```python
from build123d import *

# Parameters (mm, degrees)
CYLINDER_R           = 1.75
CYLINDER_DEPTH       = 10
CYLINDER001_R        = 4.25
CYLINDER001_DEPTH    = 8
CLONE001_ROLL_ANGLE  = 90
CLONE001_PITCH_ANGLE = -45


with BuildPart() as spacer_hole_cylinder:
    # Cylinder → Cylinder (new body)
    with BuildSketch(Plane.XY.offset(-1)):
        Circle(CYLINDER_R)
    extrude(amount=CYLINDER_DEPTH)


with BuildPart() as x_motor_spacer_top:
    # Cylinder001 → Cylinder001 (new body)
    with BuildSketch(Plane.XY):
        Circle(CYLINDER001_R)
    extrude(amount=CYLINDER001_DEPTH)

    # Cut002: cut spacer-hole-cylinder
    add(spacer_hole_cylinder.part, mode=Mode.SUBTRACT)


with BuildPart() as x_motor_spacer_top_1:
    # Clone001 roll: moved
    add(x_motor_spacer_top.part.rotate(Axis((0, 0, 0), (1, 0, 0)), CLONE001_ROLL_ANGLE))


with BuildPart() as x_motor_spacer_top_2:
    # Clone001 pitch: moved
    add(x_motor_spacer_top_1.part.rotate(Axis((0, 0, 0), (0, 1, 0)), CLONE001_PITCH_ANGLE))


with BuildPart() as x_motor_spacer_top_3:
    # Clone001 placement: moved
    add(x_motor_spacer_top_2.part.moved(Location((-49.5, 1, 41.384776))))


solid = x_motor_spacer_top_3.part
```
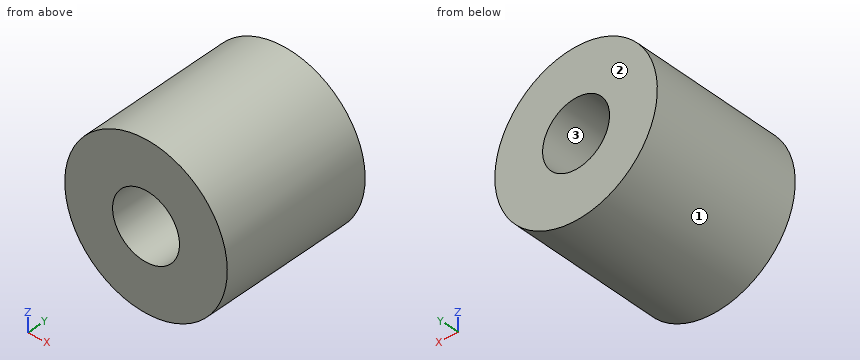
Read the model definition and answer for the solid it produces. Units are mm, in the model's axes. Face numbers are marked on the shaded views. Coordinates: 2 decimals unless noted, no trailing zeros. Loops run counter-clockwise (first coordinate to the right, second up) from the corner with the lowest first, then second, coordinate; pieces in that order, holes last. Notation, with made-up numbers: (34, -24) - (45, -24) arc R29 cw to (45, 6) - close; hole circle Ø5 at (86, 82). An arc over 180 degrees is marked (long way). Answer in a Markdown table with one row per item.
1. Find section A-A, the plane x = -49.5. Write down the section's boundary in (y, z).
Conclusion:
| item | result |
|---|---|
| outline | (-7, 37.13) - (1, 37.13) - (1, 39.63) - (-7, 39.63) - close; (-7, 43.13) - (1, 43.13) - (1, 45.63) - (-7, 45.63) - close |
2. Find section C-C, the plane y = -0.5. Write down the section's boundary in (x, z), then the cut area to 3 significant figures.
Conclusion:
| item | result |
|---|---|
| outline | circle Ø8.5 at (-49.5, 41.38); hole circle Ø3.5 at (-49.5, 41.38) |
| area | 47.1 mm² |
3. Find section B-B, the plane x = -51. Write down the section's boundary in (y, z), then the cut area to 3 significant figures.
Conclusion:
| item | result |
|---|---|
| outline | (-7, 37.41) - (1, 37.41) - (1, 40.48) - (-7, 40.48) - close; (-7, 42.29) - (1, 42.29) - (1, 45.36) - (-7, 45.36) - close |
| area | 49.2 mm² |
4. Straight lines are drawn through the part: line 1 (Z direction, x = -49.5, y = -2.75); line 2 (Z direction, x = -50.75, y = -4.75); line 3 (X direction, y = -5.5, z = 40). For each, find the intervals that lie inside material, in ascending order.
Conclusion:
| item | result |
|---|---|
| line 1 | z = 37.13 to 39.63, 43.13 to 45.63 |
| line 2 | z = 37.32 to 40.16, 42.61 to 45.45 |
| line 3 | x = -53.52 to -50.57, -48.43 to -45.48 |
5. Find section D-D, the plane x = -47. Write down the section's boundary in (y, z), then the cut area to 3 significant figures.
Conclusion:
| item | result |
|---|---|
| outline | (-7, 37.95) - (1, 37.95) - (1, 44.82) - (-7, 44.82) - close |
| area | 55.0 mm² |
6. Given pin 1 (2 mm diameter, centred on x = -49.5, z = 41.38, fed in from -Y); pin 2 (1 mm diameter, centred on x = -46, y = -5, fed in from +Z), each flat-ended and moving along its own axis, determine where each tip first touches the part or whether it passes through.
Conclusion:
| item | result |
|---|---|
| pin 1 | passes through |
| pin 2 | stops at z = 44.4 |
7. Determine the mould class of the marked faces 1, 2 and 3 for opening direction X: +X half, -X half, draft (parallel to the pull), parting line (faces both ways), or undercut.
Conclusion:
| item | result |
|---|---|
| face 1 | parting line |
| face 2 | draft |
| face 3 | undercut |
